```python
from build123d import *

# Parameters (mm, degrees)
BOSS_EXTRUDE1_DEPTH  = 50
M8_CLEARANCE_HOLE1_D = 9
SKETCH7_W            = 5
SKETCH7_H            = 30
BOSS_EXTRUDE4_DEPTH  = 30
SKETCH9_R            = 2.5
CUT_EXTRUDE1_DEPTH   = 88.007183611
SKETCH11_R           = 2
CUT_EXTRUDE2_DEPTH   = 72.414284285
BOSS_EXTRUDE7_DEPTH  = 5
FILLET4_R            = 5


with BuildPart() as part:
    # Sketch2 → Boss-Extrude1 (new, symmetric)
    with BuildSketch(Plane(origin=(0, 0, 0), x_dir=(0, 0, -1), z_dir=(1, 0, 0))):
        Polygon((0, 0), (-24.748737342, 24.748737342), (-28.284271247, 21.213203436), (0, -7.071067812), (28.284271247, 21.213203436), (24.748737342, 24.748737342), align=None)
    extrude(amount=BOSS_EXTRUDE1_DEPTH, both=True)

    # M8 Clearance Hole1 (through all)
    with Locations(Plane(origin=(0, 0, 0), x_dir=(1, 0, 0), z_dir=(0, 0.7071067811865489, 0.7071067811865461))):
        with Locations((0, 10)):
            Hole(M8_CLEARANCE_HOLE1_D / 2)

    # Sketch7 → Boss-Extrude4 (add)
    with BuildSketch(Plane(origin=(0, -3.535533906, -3.535533906), x_dir=(1, 0, 0), z_dir=(0, -0.7071067811865479, -0.7071067811865471))):
        with Locations((18, -10)):
            Rectangle(SKETCH7_W, SKETCH7_H)
        with Locations((-18, -10)):
            Rectangle(SKETCH7_W, SKETCH7_H)
    extrude(amount=BOSS_EXTRUDE4_DEPTH)

    # Sketch9 → Cut-Extrude1 (cut, through all)
    with BuildSketch(Plane(origin=(20.5, 0, 0), x_dir=(0, 0, -1), z_dir=(1, 0, 0))):
        with Locations((21.213203436, -7.071067812)):
            Circle(SKETCH9_R)
    extrude(amount=-CUT_EXTRUDE1_DEPTH, mode=Mode.SUBTRACT)

    # Sketch11 → Cut-Extrude2 (cut, through all)
    with BuildSketch(Plane(origin=(0, 0, 0), x_dir=(1, 0, 0), z_dir=(0, 0.7071067811865477, 0.7071067811865474))):
        with Locations(Location((-40, 30, 0), (0, 0, 270))):
            Circle(SKETCH11_R)
        with Locations(Location((-40, 5, 0), (0, 0, 270))):
            Circle(SKETCH11_R)
        with Locations(Location((40, 30, 0), (0, 0, 270))):
            Circle(SKETCH11_R)
        with Locations(Location((40, 5, 0), (0, 0, 270))):
            Circle(SKETCH11_R)
    cut_extrude2 = extrude(amount=-CUT_EXTRUDE2_DEPTH, mode=Mode.SUBTRACT)

    # Mirror1: Cut-Extrude2 across plane
    add(cut_extrude2.mirror(Plane.XY), mode=Mode.SUBTRACT)

    # Sketch12 → Boss-Extrude7 (add)
    with BuildSketch(Plane(origin=(0, -3.535533906, 3.535533906), x_dir=(1, 0, 0), z_dir=(0, 0.7071067811865475, -0.7071067811865477))):
        Polygon((-50, 5), (-20.5, 35), (-20.5, 5), align=None)
        Polygon((20.5, 5), (20.5, 35), (50, 5), align=None)
    extrude(amount=BOSS_EXTRUDE7_DEPTH)

    # Fillet4
    fillet4_edges = [part.edges().sort_by_distance(p)[0] for p in [
        (50, 22.980970389, 26.516504294),
        (50, 22.980970389, -26.516504294),
        (18, -7.071067812, -42.426406871),
        (-18, -7.071067812, -42.426406871),
        (-50, 22.980970389, -26.516504294),
        (-50, 22.980970389, 26.516504294),
    ]]
    fillet(fillet4_edges, radius=FILLET4_R)


solid = part.part
```
The model under review builds one solid part; all positions refer to its coordinate system, in mm. A direction names the side the tool comes from. Round coordinates to 2 decimals unless told otherwise and drop trailing zeros. Loops run counter-clockwise (first coordinate to the right, second up) from the corner with the lowest first, then second, coordinate; pieces in that order, holes last.
1) Tool access review of faces 1 (the face through (1, 13, -13)), 2 (the face through (-28, -10, -10)), 3 (the face through (-18, -19.6, -29.9)): name each direction out of +Z, -Z, +X, -X, +Y, -Y from which nothing blocks a thin tool from reaching the whole face with its end or side.
Values follow:
face 1: +X, -X, +Y
face 2: -Z, -X
face 3: -Z, +X, -X, -Y
2) The part is to be moulded in two halves that separate along X. For faces 4 (the face through (-15.5, -9, -24)), 5 (the face through (0.6, 23, 26.5)), 6 (the face through (50, 3, -4)), say which applies: pulls with the +X half, pulls with the -X half, needs draft (parallel to the pull), parting line crosses it, or undercut.
Values follow:
face 4: undercut
face 5: needs draft
face 6: pulls with the +X half
3) Consider section D-D on z = 17. State the section outline as (x, y) points, then the cut area to 3 significant figures.
Values follow:
outline: (-50, 9.93) - (50, 9.93) - (50, 17) - (-50, 17) - close
area: 707 mm2
4) Consider section B-B on x = 35. State the section outline as (y, z) points, then the cut area to 3 significant figures.
Values follow:
outline: (-17.86, -10.79) - (-14.32, -14.32) - (-3.54, -3.54) - (21.21, -28.28) - (24.75, -24.75) - (0, 0) - (24.75, 24.75) - (21.21, 28.28) - close
area: 451 mm2
5) Consider section A-A on y = -22. State the section outline as (x, z) points.
Values follow:
outline: (-29.24, -14.93) - (-24.32, -22) - (-20.5, -22) - (-20.5, -27.5) - (-15.5, -27.5) - (-15.5, -14.93) - close; (15.5, -27.5) - (20.5, -27.5) - (20.5, -22) - (24.32, -22) - (29.24, -14.93) - (15.5, -14.93) - close
6) Wall thickness on line 1 along X through (y, z) = (-13.5, -29.5); line 2 along Y through (x, z) = (-38.5, -5.5); line 3 along Z through (x, y) = (8.5, 8): over which ranges is each line inside the solid? List them lowest first.
Values follow:
line 1: x = -20.5 to -15.5, 15.5 to 20.5
line 2: y = -12.57 to -5.5, -1.57 to -0.3, 3.44 to 5.5
line 3: z = -15.07 to -8, 8 to 15.07
7) Clearance check with flat-ended pins moving along their axes: P1, Ø3, axis at x = -38.5, y = -11.5, coming from the +Z side; P2, Ø1, axis at x = 38, y = -2.5, coming from the -Z side; P3, Ø3, axis at x = 15, z = 14.5, coming from the +Y side. State where each tip first meets the part, or that it passes through.
Values follow:
P1: stops at z = -2.93
P2: stops at z = -5.07
P3: stops at y = 16
8) Consider section C-C on y = 13. State the section outline as (x, z) points.
Values follow:
outline: (-50, -20.07) - (-20.5, -20.07) - (-20.5, -22.36) - (-15.5, -22.36) - (-15.5, -20.07) - (15.5, -20.07) - (15.5, -22.36) - (20.5, -22.36) - (20.5, -20.07) - (50, -20.07) - (50, -13) - (-50, -13) - close; (-50, 13) - (50, 13) - (50, 20.07) - (-50, 20.07) - close
